Job drawing, mm, ordinate dimensions from the low corner. One solid piece. A direction names the side the tool comes from. Give positions to 0.01 mm unless a question says otherwise; leave off trailing zeros. Order: outer loops, then holes, each group sorted by start corner. A loop starts at its lowest first (then second) coordinate and runs counter-clockwise, first axis right, second up.
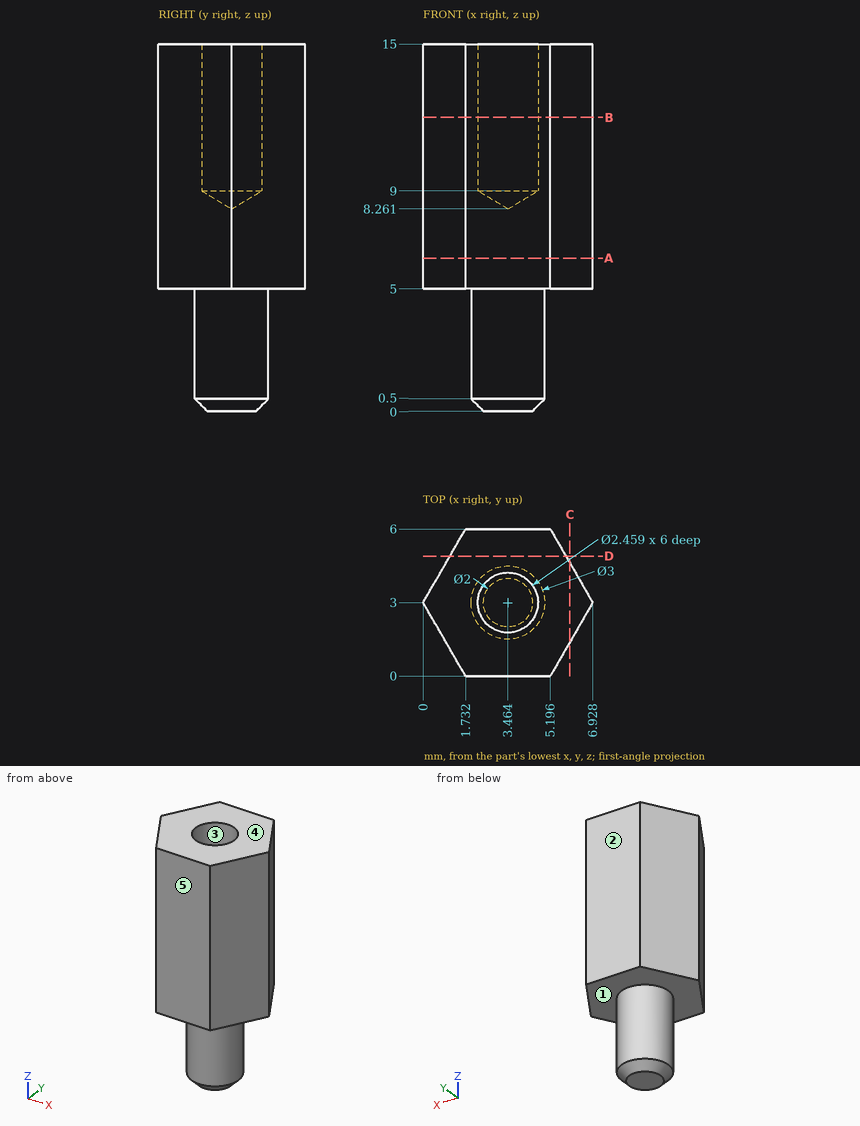
Item 1: Drop flat-ended pins along their axis: P1, Ø2, axis at x = 3.46, y = 3, coming from the +Z side (1 decimal); P2, Ø3, axis at x = 6, y = 3.5, coming from the -Z side (1 decimal). Give the stop position or say it passes through.
Item 2: Which spindle directions (+Z, -Z, +X, -X, +Y, -Y) get a long thin tool onto all of the face, cutting with end or side? Do the marked faces 1 and 2. Say none if no direction does.
Item 3: Pull direction Y, two halves, no side cores. Call the marked faces 3, 4 and 5: released by +Y, released by -Y, zero draft, split by the parting line, or undercut.
Item 4: Band-saw the part on B-B on z = 12. List the corners of the cut face in (x, y).
Item 5: Band-saw the part on C-C on x = 6. List the corners of the cut face in (y, z).
Item 6: Band-saw the part on D-D on y = 4.9. List the corners of the cut face in (x, z).
Item 7: Drill centre lines: probe 1 along Z at (x, y) = (5, 2.5); probe 2 along X at (y, z) = (1.95, 12.25) (1 decimal); probe 3 along X at (y, z) = (2.85, 10.25) (1 decimal). Where is each one in solid material? Low to high.
Item 8: Band-saw the part on A-A on z = 6.25. List the corners of the cut face in (x, y).
Working result:
1. P1: stops at z = 8.9
1. P2: stops at z = 0.1
2. face 1: -Z
2. face 2: +Z, -Z, +X, -X, +Y
3. face 3: undercut
3. face 4: zero draft
3. face 5: released by -Y
4. outline: (0, 3) - (1.73, 0) - (5.2, 0) - (6.93, 3) - (5.2, 6) - (1.73, 6) - close; hole circle Ø2.46 at (3.46, 3)
5. outline: (1.39, 5) - (4.61, 5) - (4.61, 15) - (1.39, 15) - close
6. outline: (1.1, 5) - (5.83, 5) - (5.83, 15) - (1.1, 15) - close
7. probe 1: z = 5 to 15
7. probe 2: x = 0.6 to 2.8, 4.1 to 6.3
7. probe 3: x = 0.1 to 2.2, 4.7 to 6.8
8. outline: (0, 3) - (1.73, 0) - (5.2, 0) - (6.93, 3) - (5.2, 6) - (1.73, 6) - close
